Could you check a few things on this drawing? It's one solid part, dimensions in mm from its lowest x, y, z. A direction names the side the tool comes from. Give positions to 0.01 mm unless a question says otherwise; leave off trailing zeros. Loops run counter-clockwise (first coordinate to the right, second up) from the corner with the lowest first, then second, coordinate; pieces in that order, holes last. Notation, with made-up numbers: (-12, -30) - (14, -30) arc R15 cw to (14, -8) - close; hole circle Ø4 at (78, 7.5). An arc over 180 degrees is marked (long way). Use a Markdown table: item, result.
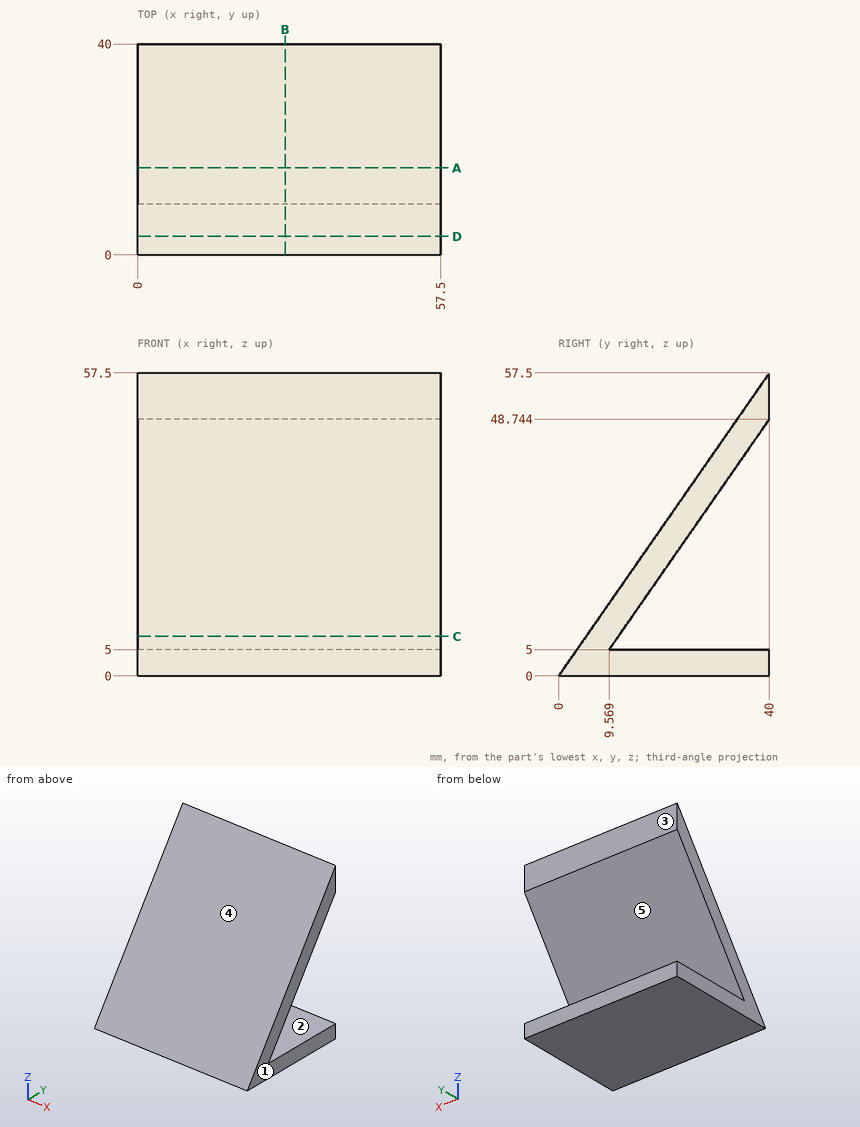
(1) Suppose I cut it at D-D on y = 3.5. Write out the boundary of the cut face in (x, z).
A:
| item | result |
|---|---|
| outline | (0, 0) - (57.5, 0) - (57.5, 5.03) - (0, 5.03) - close |
(2) We'd pull the mould along Z, two halves only. Please class the marked faces 3, 4 and 5: pulls with the +Z half, pulls with the -Z half, needs draft (parallel to the pull), parting line crosses it, or undercut.
A:
| item | result |
|---|---|
| face 3 | needs draft |
| face 4 | pulls with the +Z half |
| face 5 | undercut |
(3) Will these pins go through, and if not, where does the flat tip stop? pin 1 (15 mm diameter, centred on x = 41.5, y = 30, fed in from +Z) (1 decimal); pin 2 (4 mm diameter, centred on y = 18, z = 13, fed in from +X); pin 3 (12 mm diameter, centred on x = 44.5, y = 6.5, fed in from +Z); pin 4 (12 mm diameter, centred on x = 17, z = 26.5, fed in from +Y).
A:
| item | result |
|---|---|
| pin 1 | z = 53.9 |
| pin 2 | through |
| pin 3 | z = 17.97 |
| pin 4 | y = 28.7 |
(4) If I drill on line 1 (Z direction, x = 54.5, y = 30.5) (1 decimal); line 2 (Z direction, x = 9, y = 16) (1 decimal); line 3 (Y direction, x = 4.5, z = 49.5) (1 decimal), over which ranges is the centre line in solid material (lowest first)?
A:
| item | result |
|---|---|
| line 1 | 0 to 5, 35.1 to 43.8 |
| line 2 | 0 to 5, 14.2 to 23 |
| line 3 | 34.4 to 40 |
(5) On a 3-axis mill with a long thin cutter (end or side, diameter ignored), from which of +Z, -Z, +X, -X, +Y, -Y can I reach the whole of each face in a straight line? I mean the marked faces 1 and 2. Say none if no direction works.
A:
| item | result |
|---|---|
| face 1 | +Z, -Z, +X, +Y, -Y |
| face 2 | +X, -X, +Y |
(6) Suppose I cut it at A-A on y = 16.5. Write out the boundary of the cut face in (x, z).
A:
| item | result |
|---|---|
| outline | (0, 0) - (57.5, 0) - (57.5, 5) - (0, 5) - close; (0, 14.96) - (57.5, 14.96) - (57.5, 23.72) - (0, 23.72) - close |
(7) Suppose I cut it at C-C on z = 7.5. Write out the boundary of the cut face in (x, y), plus the area to 3 significant figures.
A:
| item | result |
|---|---|
| outline | (0, 5.22) - (57.5, 5.22) - (57.5, 11.31) - (0, 11.31) - close |
| area | 350 mm2 |
(8) Suppose I cut it at B-B on x = 28. Write out the boundary of the cut face in (y, z) (1 decimal).
A:
| item | result |
|---|---|
| outline | (0, 0) - (40, 0) - (40, 5) - (9.6, 5) - (40, 48.7) - (40, 57.5) - close |
